from build123d import *

# Parameters (mm, degrees)
BOSS_EXTRU_1_DEPTH      = 6
ESQUISSE2_R             = 3.65
ESQUISSE2_R_2           = 1.4
ENL_V_MAT_EXTRU_1_DEPTH = 6


with BuildPart() as part:
    # Esquisse1 → Boss.-Extru.1 (new body)
    with BuildSketch(Plane.XY):
        with BuildLine():
            Line((-5, 18.927916642), (5, 18.927916642))
            Line((5, 18.927916642), (5, -11.072083358))
            ThreePointArc((5, -11.072083358), (0, -22.971062844), (-5, -11.072083358))
            Line((-5, -11.072083358), (-5, 18.927916642))
        make_face()
    extrude(amount=BOSS_EXTRU_1_DEPTH)

    # Esquisse2 → Enlèv. mat.-Extru.1 (cut)
    with BuildSketch(Plane(origin=(0, 0, 0), x_dir=(-1, 0, 0), z_dir=(0, 0, -1))):
        with Locations((0, -15.799586654)):
            Circle(ESQUISSE2_R)
        with Locations((0, -1.072083358)):
            Circle(ESQUISSE2_R_2)
        with Locations((0, 13.927916642)):
            Circle(ESQUISSE2_R_2)
    extrude(amount=-ENL_V_MAT_EXTRU_1_DEPTH, mode=Mode.SUBTRACT)


solid = part.part
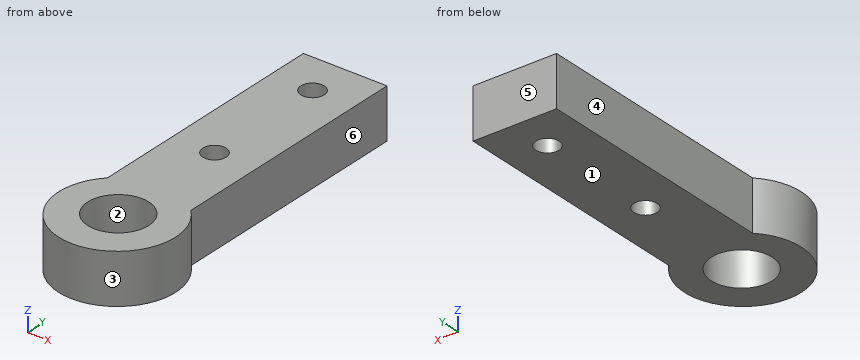
Here's how the part is built. I have some questions about the finished solid (model axes, mm). Face numbers are marked on the shaded views. A direction names the side the tool comes from. Round coordinates to 2 decimals unless told otherwise and drop trailing zeros. Order: outer loops, then holes, each group sorted by start corner. A loop starts at its lowest first (then second) coordinate and runs counter-clockwise, first axis right, second up. Notation, with made-up numbers: M 83,21.25 L 113,21.25 A30 ccw 113,47.25 Z; hole C -4.5,55.5 d7. An arc over 180 degrees is marked long. One line per question, with ' | ' between items.
1) I'm going to push flat-ended pins straight in: pin 1 Ø1.8 at (y, z) = (-3, 1.5) entering from -X; pin 2 Ø2 at (y, z) = (9, 1) entering from +X; pin 3 Ø6.5 at (x, y) = (0, -15.8) entering from -Z; pin 4 Ø2 at (y, z) = (-17.5, 5) entering from -X. Where does each tip first touch, or does it pass through?
Checked values:
pin 1: stops at x = -5 | pin 2: stops at x = 5 | pin 3: passes through | pin 4: stops at x = -6.98
2) Imagine slicing it at B-B, the plane y = 13.5. Write out the boundary of the cut face in (x, z), plus the area to 3 significant figures.
Checked values:
outline: M -5,0 L -1.33,0 L -1.33,6 L -5,6 Z; M 1.33,0 L 5,0 L 5,6 L 1.33,6 Z | area: 44.0 mm²
3) On a 3-axis mill with a long thin cutter (end or side, diameter ignored), from which of +Z, -Z, +X, -X, +Y, -Y can I reach the whole of each face in a straight line? I mean the marked faces 4, 5 and 6. Say none if no direction works.
Checked values:
face 4: +Z, -Z, -X, +Y | face 5: +Z, -Z, +X, -X, +Y | face 6: +Z, -Z, +X, +Y
4) We'd pull the mould along Y, two halves only. Please class the marked faces 1, 2 and 3: released by +Y, released by -Y, zero draft, split by the parting line, or undercut.
Checked values:
face 1: zero draft | face 2: undercut | face 3: split by the parting line
5) I need wall thicknesses on line 1 (Y direction, x = 0, z = 2); line 2 (X direction, y = -1, z = 1.15); line 3 (Y direction, x = 0.25, z = 4.8). Which ranges of each line are inside material? Lowest first, please.
Checked values:
line 1: y = -22.97 to -19.45, -12.15 to -2.47, 0.33 to 12.53, 15.33 to 18.93 | line 2: x = -5 to -1.4, 1.4 to 5 | line 3: y = -22.97 to -19.44, -12.16 to -2.45, 0.31 to 12.55, 15.31 to 18.93
6) Imagine slicing it at A-A, the plane x = 0. Write out the boundary of the cut face in (y, z).
Checked values:
outline: M -22.97,0 L -19.45,0 L -19.45,6 L -22.97,6 Z; M -12.15,0 L -2.47,0 L -2.47,6 L -12.15,6 Z; M 0.33,0 L 12.53,0 L 12.53,6 L 0.33,6 Z; M 15.33,0 L 18.93,0 L 18.93,6 L 15.33,6 Z
7) Imagine slicing it at D-D, the plane x = 2. Write out the boundary of the cut face in (y, z).
Checked values:
outline: M -22.68,0 L -18.85,0 L -18.85,6 L -22.68,6 Z; M -12.75,0 L 18.93,0 L 18.93,6 L -12.75,6 Z
8) Imagine slicing it at C-C, the plane z = 1.4. Write out the boundary of the cut face in (x, y).
Checked values:
outline: M -5,-11.07 A7 ccw long 5,-11.07 L 5,18.93 L -5,18.93 Z; hole C 0,-15.8 d7.3; hole C 0,-1.07 d2.8; hole C 0,13.93 d2.8
